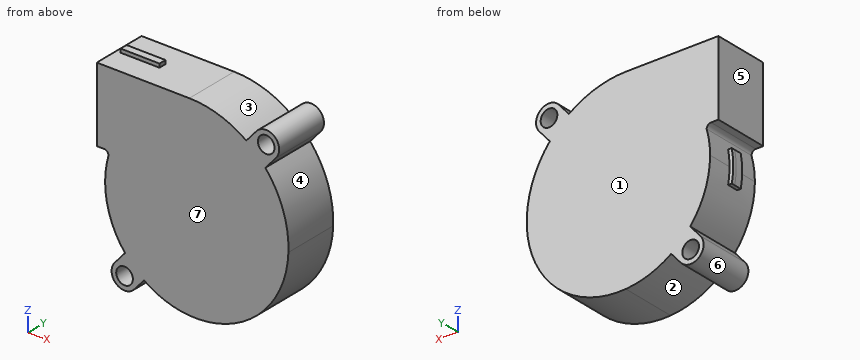
from build123d import *

# Parameters (mm, degrees)
SKETCH1_R                = 2.25
BOSS_EXTRUDE1_DEPTH      = 7.5
BOSS_EXTRUDE1_DEPTH_BACK = 7.5
BOSS_EXTRUDE2_DEPTH      = 1
BOSS_EXTRUDE2_DEPTH_BACK = 2
SKETCH3_W                = 10.5
SKETCH3_H                = 1
BOSS_EXTRUDE3_DEPTH      = 1
BOSS_EXTRUDE3_DEPTH_BACK = 1


with BuildPart() as part:
    # Sketch1 → Boss-Extrude1 (new body, two sides)
    with BuildSketch(Plane(origin=(0, 0, 0), x_dir=(1, 0, 0), z_dir=(0, 1, 0))) as boss_extrude1_sk:
        with BuildLine():
            Line((0, -27.75), (-25, -27.75))
            Line((-25, -27.75), (-25, -7.75))
            Line((-25, -7.75), (-23, -7.75))
            ThreePointArc((-23, -7.75), (-22.173642142, -7.407711368), (-21.83135351, -6.58135351))
            ThreePointArc((-21.83135351, -6.58135351), (-22.519230493, -3.322579021), (-22.75, 0))
            ThreePointArc((-22.75, 0), (-21.367673649, 8.078905587), (-17.377967793, 15.238639437))
            Line((-17.377967793, 15.238639437), (-20.154237836, 18.468548377))
            ThreePointArc((-20.154237836, 18.468548377), (-19.781451623, 23.404237836), (-14.845762164, 23.031451623))
            Line((-14.845762164, 23.031451623), (-12.244288682, 20.004900775))
            ThreePointArc((-12.244288682, 20.004900775), (-6.410360065, 22.958761116), (0, 24.25))
            ThreePointArc((0, 24.25), (18.502982119, 17.781640069), (26.75, 0))
            ThreePointArc((26.75, 0), (25.310000225, -9.634196337), (20.525571791, -18.119512063))
            Line((20.525571791, -18.119512063), (23.404237836, -21.468548377))
            ThreePointArc((23.404237836, -21.468548377), (23.031451623, -26.404237836), (18.095762164, -26.031451623))
            Line((18.095762164, -26.031451623), (15.372148216, -22.862802716))
            ThreePointArc((15.372148216, -22.862802716), (8.06198842, -26.488798996), (0, -27.75))
        make_face()
        with Locations((-17.5, 20.75)):
            Circle(SKETCH1_R, mode=Mode.SUBTRACT)
        with Locations((20.75, -23.75)):
            Circle(SKETCH1_R, mode=Mode.SUBTRACT)
    extrude(amount=BOSS_EXTRUDE1_DEPTH)
    extrude(boss_extrude1_sk.sketch, amount=-BOSS_EXTRUDE1_DEPTH_BACK)

    # Sketch2 → Boss-Extrude2 (add, two sides)
    with BuildSketch(Plane(origin=(0, 0, 0), x_dir=(1, 0, 0), z_dir=(0, 1, 0))) as boss_extrude2_sk:
        with BuildLine():
            Line((-23.375448552, 4.25), (-22.375448552, 4.25))
            Line((-22.375448552, 4.25), (-20.476060309, 3.242316336))
            Line((-20.476060309, 3.242316336), (-20.106924084, -2.963786455))
            Line((-20.106924084, -2.963786455), (-22.3712513, -4.25))
            Line((-22.3712513, -4.25), (-23.3712513, -4.25))
            add(Edge.make_bspline(
                [(-23.3712513, -4.25), (-24.126649893, -0.000369077), (-23.375448552, 4.25)],
                knots=[0, 0, 0, 1, 1, 1], degree=2))
        make_face()
    extrude(amount=BOSS_EXTRUDE2_DEPTH)
    extrude(boss_extrude2_sk.sketch, amount=-BOSS_EXTRUDE2_DEPTH_BACK)

    # Sketch3 → Boss-Extrude3 (add, two sides)
    with BuildSketch(Plane(origin=(0, 0, 0), x_dir=(1, 0, 0), z_dir=(0, 1, 0))) as boss_extrude3_sk:
        with Locations((-18.55, -28.25)):
            Rectangle(SKETCH3_W, SKETCH3_H)
    extrude(amount=BOSS_EXTRUDE3_DEPTH)
    extrude(boss_extrude3_sk.sketch, amount=-BOSS_EXTRUDE3_DEPTH_BACK)


solid = part.part
Can you work these out from the model? Positions are in its coordinate system, mm. Face numbers are marked on the shaded views. A direction names the side the tool comes from. Coordinates: 2 decimals unless noted, no trailing zeros. Loops run counter-clockwise (first coordinate to the right, second up) from the corner with the lowest first, then second, coordinate; pieces in that order, holes last. Notation, with made-up numbers: (-28.75, 80) - (-19.75, 80) arc R16 ccw to (-19.75, 111) - close; hole circle Ø3 at (48, 13). An arc over 180 degrees is marked (long way). Answer as a JSON object with one key per item and string values. Group by question number.
Item 1: If we section it at B-B (z = -20.75): List the corners of the cut face in (x, y) for me.
Item 2: If we section it at C-C (z = 23.75): List the corners of the cut face in (x, y) for me.
Item 3: On a 3-axis mill with a long thin cutter (end or side, diameter ignored), from which of +Z, -Z, +X, -X, +Y, -Y can I reach the whole of each face in a straight line? I mean the marked faces 1, 2 and 3. Say none if no direction works.
Item 4: If we mould it in two halves opening along X, with no side actions, what happens to the marked faces 4, 5, 6 and 7? For each: released by +X, released by -X, zero draft, split by the parting line, or undercut.
Item 5: For pin 1 (7.5 mm diameter, centred on x = -8, y = 3, fed in from +Z); pin 2 (1.5 mm diameter, centred on y = -1.5, z = -5, fed in from +X); pin 3 (1 mm diameter, centred on x = -24.5, y = 1, fed in from -Z), each with a flat end and sliding along its axis, tell me the tip position at first contact or that it passes through.
Item 6: If we section it at D-D (z = 16.5): List the corners of the cut face in (x, y) for me, plus the area to 3 significant figures.
Item 7: If we section it at A-A (y = 6.5): List the corners of the cut face in (x, z) for me, plus the area to 3 significant figures.
Item 8: If I drill on L1, parallel to Z at x = -17.5, y = 4.5; L2, parallel to Z at x = -18, y = -4; L3, parallel to X at y = -1.5, z = -20.75, over which ranges is the centre line in solid material (lowest first)? Write a range as from..to.
Returned:
{
 "1": {"outline": "(-21, -7.5) - (-19.75, -7.5) - (-19.75, 7.5) - (-21, 7.5) - close; (-15.25, -7.5) - (-12.88, -7.5) - (-12.88, 7.5) - (-15.25, 7.5) - close; (-11.1, -7.5) - (14.49, -7.5) - (14.49, 7.5) - (-11.1, 7.5) - close"},
 "2": {"outline": "(-25, -7.5) - (14.03, -7.5) - (14.03, 7.5) - (-25, 7.5) - close; (16.13, -7.5) - (18.5, -7.5) - (18.5, 7.5) - (16.13, 7.5) - close; (23, -7.5) - (24.25, -7.5) - (24.25, 7.5) - (23, 7.5) - close"},
 "3": {"face 1": "+Z, -Z, +X, -X, +Y", "face 2": "-Z, +Y, -Y", "face 3": "+Z, +Y, -Y"},
 "4": {"face 4": "released by +X", "face 5": "released by -X", "face 6": "undercut", "face 7": "zero draft"},
 "5": {"pin 1": "stops at z = 27.75", "pin 2": "stops at x = 26.24", "pin 3": "stops at z = 7.75"},
 "6": {"outline": "(-25, -7.5) - (21.78, -7.5) - (21.78, 7.5) - (-25, 7.5) - close", "area": "702 mm²"},
 "7": {"outline": "(-25, 7.75) - (-23, 7.75) arc R1.17 cw to (-21.83, 6.58) arc R24.03 ccw to (-22.75, 0) arc R24.3 ccw to (-17.38, -15.24) - (-20.15, -18.47) arc R3.5 ccw to (-14.85, -23.03) - (-12.24, -20) arc R24.3 ccw to (0, -24.25) arc R25.16 ccw to (26.75, 0) arc R26.83 ccw to (20.53, 18.12) - (23.4, 21.47) arc R3.5 ccw to (18.1, 26.03) - (15.37, 22.86) arc R26.83 ccw to (0, 27.75) - (-25, 27.75) - close; hole circle Ø4.5 at (-17.5, -20.75); hole circle Ø4.5 at (20.75, 23.75)", "area": "2,270 mm²"},
 "8": {"L1": "z = -24.25..-23, -18.5..-15.38, -15.09..27.75", "L2": "z = -24.21..-22.94, -18.56..-15.96, -14.43..27.75", "L3": "x = -21..-19.75, -15.25..-12.88, -11.1..14.49"}
}
